Input: dimensioned drawing with shaded views. Units: mm. Origin: part minimum x, y, z. A direction names the side the tool comes from. Give positions to 0.01 mm unless a question says otherwise; leave off trailing zeros. Write each loop counter-clockwise with the first axis right and the second up, starting at its lowest first coordinate (ties: lowest second). Pieces come first, ordered by that corner, then holes.
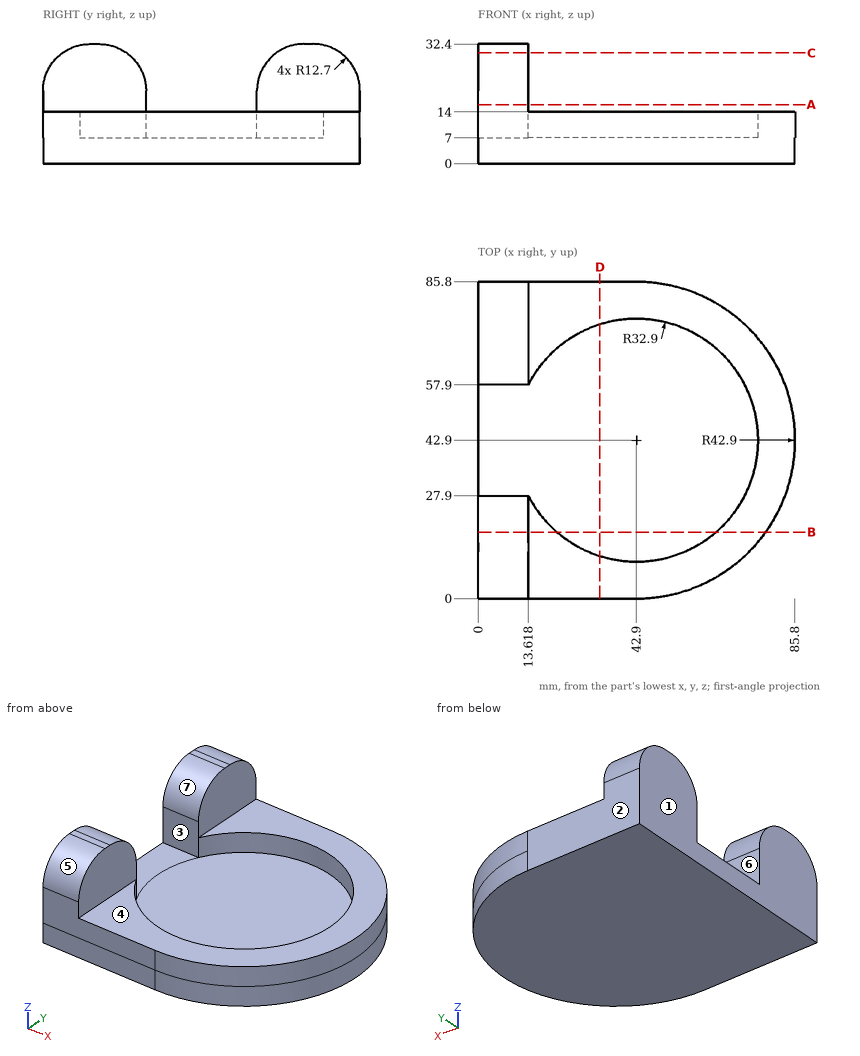
Item 1: Reachability of the marked faces 4, 5, 6 and 7 from +Z, -Z, +X, -X, +Y, -Y: full face, straight path, thin tool, end or side. Return the list, or none.
Found:
face 4: +Z, +X, +Y, -Y
face 5: +Z, +X, -X, -Y
face 6: +Z, -X
face 7: +Z, +X, -X
Item 2: Section B-B, the plane y = 18. Return the cut outline in (x, z) (1 decimal).
Found:
outline: (0, 0) - (77.8, 0) - (77.8, 14) - (64.4, 14) - (64.4, 7) - (21.4, 7) - (21.4, 14) - (13.6, 14) - (13.6, 32.1) - (0, 32.1) - close
Item 3: Section C-C, the plane z = 30. Return the cut outline in (x, y).
Found:
outline: (0, 5.27) - (13.62, 5.27) - (13.62, 22.63) - (0, 22.63) - close; (0, 63.17) - (13.62, 63.17) - (13.62, 80.53) - (0, 80.53) - close
Item 4: Section A-A, the plane z = 16. Return the cut outline in (x, y), plus the area to 3 significant figures.
Found:
outline: (0, 0) - (13.62, 0) - (13.62, 27.9) - (0, 27.9) - close; (0, 57.9) - (13.62, 57.9) - (13.62, 85.8) - (0, 85.8) - close
area: 760 mm2
Item 5: Line query: L1, parallel to Y at x = 13, z = 17.5; L2, parallel to Y at x = 44, z = 9.5 (1 decimal); L3, parallel to Z at x = 58, y = 20.5. Output: solid intervals per line, ascending.
Found:
L1: y = 0 to 27.9, 57.9 to 85.8
L2: y = 0 to 10, 75.8 to 85.8
L3: z = 0 to 7
Item 6: Pin query (flat end, axial travel): pin 1 Ø12 at (y, z) = (27.5, 22.5) entering from +X; pin 2 Ø4 at (x, y) = (56, 28.5) entering from +Z; pin 3 Ø1 at (x, z) = (55.5, 12.5) entering from +Y. Return the tip coordinate at first contact, or that it passes through.
Found:
pin 1: stops at x = 13.62
pin 2: stops at z = 7
pin 3: stops at y = 84.06
Item 7: Section D-D, the plane x = 33. Return the cut outline in (y, z) (1 decimal).
Found:
outline: (0, 0) - (85.8, 0) - (85.8, 14) - (74.3, 14) - (74.3, 7) - (11.5, 7) - (11.5, 14) - (0, 14) - close
Item 8: Pull-direction query (Y, two-part tool) for the marked faces 1, 2 and 3; classes: +Y half, -Y half, draft (parallel to the pull), parting line (faces both ways), or undercut.
Found:
face 1: draft
face 2: +Y half
face 3: undercut
